from build123d import *

# Parameters (mm, degrees)
BOSS_EXTRU_1_DEPTH      = 39.5
ESQUISSE3_W             = 10
ESQUISSE3_H             = 5
ENL_V_MAT_EXTRU_1_DEPTH = 51.963222033
CUT_EXTRUDE1_DEPTH      = 64.947243881
CUT_EXTRUDE1_DEPTH_BACK = 64.947243881
SKETCH1_R               = 1.6
CUT_EXTRUDE2_DEPTH      = 51.963222033
FILLET1_R               = 5


with BuildPart() as part:
    # Esquisse1 → Boss.-Extru.1 (new body)
    with BuildSketch(Plane.XY):
        Polygon((-22, 0), (22, 0), (22, 15), (26, 15), (26, -4), (-26, -4), (-26, 15), (-22, 15), align=None)
    extrude(amount=BOSS_EXTRU_1_DEPTH)

    # Esquisse3 → Enlèv. mat.-Extru.1 (cut, through all)
    with BuildSketch(Plane.XZ.offset(4)):
        with Locations((0, 7)):
            Rectangle(ESQUISSE3_W, ESQUISSE3_H)
    extrude(amount=-ENL_V_MAT_EXTRU_1_DEPTH, mode=Mode.SUBTRACT)

    # Sketch1 → Cut-Extrude1 (cut, two sides: drawn at the far end of the back side and taken through both)
    with BuildSketch(Plane(origin=(-22, 0, 0), x_dir=(0, 0, -1), z_dir=(1, 0, 0)).offset(-CUT_EXTRUDE1_DEPTH_BACK)):
        with Locations((-19.75, 6)):
            Circle(SKETCH1_R)
    extrude(amount=CUT_EXTRUDE1_DEPTH + CUT_EXTRUDE1_DEPTH_BACK, mode=Mode.SUBTRACT)

    # Sketch2 → Cut-Extrude2 (cut, through all)
    with BuildSketch(Plane.XZ.offset(4)):
        with BuildLine():
            Line((-16.9, 30.226876468), (-16.9, 15.226876468))
            ThreePointArc((-16.9, 15.226876468), (-18.5, 13.626876468), (-20.1, 15.226876468))
            Line((-20.1, 15.226876468), (-20.1, 30.226876468))
            ThreePointArc((-20.1, 30.226876468), (-18.5, 31.826876468), (-16.9, 30.226876468))
        make_face()
        with BuildLine():
            Line((20.1, 30.226876468), (20.1, 15.226876468))
            ThreePointArc((20.1, 15.226876468), (18.5, 13.626876468), (16.9, 15.226876468))
            Line((16.9, 15.226876468), (16.9, 30.226876468))
            ThreePointArc((16.9, 30.226876468), (18.5, 31.826876468), (20.1, 30.226876468))
        make_face()
    extrude(amount=-CUT_EXTRUDE2_DEPTH, mode=Mode.SUBTRACT)

    # Fillet1
    fillet1_edges = [part.edges().sort_by_distance(p)[0] for p in [
        (26, -4, 19.75),
        (-26, -4, 19.75),
    ]]
    fillet(fillet1_edges, radius=FILLET1_R)


solid = part.part
Design review of the part built by this model. Coordinates are the model's own, in mm. A direction names the side the tool comes from. Coordinates: 2 decimals unless noted, no trailing zeros. Order: outer loops, then holes, each group sorted by start corner. A loop starts at its lowest first (then second) coordinate and runs counter-clockwise, first axis right, second up. Notation, with made-up numbers: (53, 17.25) -> (69, 17.25) arc R19 ccw to (69, 50.25) -> close; hole circle Ø8 at (47, 27.25). An arc over 180 degrees is marked (long way). Use one line per item in the form item = value. Start each with the question number.
(1) Add section C-C on x = 18.5. State the section outline as (y, z) points.
(2) Add section A-A on y = 9.25. State the section outline as (x, z) points, plus the area to 3 significant figures.
(3) The part is to be moulded in two halves that separate along Z. For faces 4 (the flat face through (16.9, -2, 23)), 5 (the flat face through (5, -2, 7)), 6 (the flat face through (-24, 15, 19)), say which applies: +Z half, -Z half, draft (parallel to the pull), parting line (faces both ways), or undercut.
(4) For faces 1 (the flat face through (0, -2, 9.5)), 2 (the flat face through (0, 0, 19)), 3 (the cylindrical face through (24, 5, 21)), list the 3-axis set-ups (+Z, -Z, +X, -X, +Y, -Y) from which the entire face can be reached by the end or side of a thin tool; tool diameter is ignored.
(5) Add section D-D on z = 26. State the section outline as (x, y) points.
(6) Insertion check: pin 1 (2 mm diameter, centred on y = -2, z = 22.5, fed in from -X); pin 2 (3 mm diameter, centred on y = -3, z = 24.5, fed in from +X); pin 3 (1 mm diameter, centred on x = 3, y = 1, fed in from +Z); pin 4 (3 mm diameter, centred on x = 16, z = 33, fed in from +Y). Each pin has a flat end and moves straight along its axis. Give the tip position at first contact, or say it passes through.
(7) Add section B-B on z = 19.75. State the section outline as (x, y) points, plus the area to 3 significant figures.
(8) For probe 1 along Z at (x, y) = (24.15, 6); probe 2 along X at (y, z) = (12, 34); probe 3 along X at (y, z) = (-2.75, 28), list the stretches that pass through material, from the lowest coordinate up.
Answer block:
q1.outline = (-4, 0) -> (0, 0) -> (0, 13.63) -> (-4, 13.63) -> close; (-4, 31.83) -> (0, 31.83) -> (0, 39.5) -> (-4, 39.5) -> close
q2.outline = (-26, 0) -> (-22, 0) -> (-22, 39.5) -> (-26, 39.5) -> close; (22, 0) -> (26, 0) -> (26, 39.5) -> (22, 39.5) -> close
q2.area = 316 mm²
q3.face_4 = undercut
q3.face_5 = undercut
q3.face_6 = draft
q4.face_1 = +Y, -Y
q4.face_2 = +Z, -Z, +Y
q4.face_3 = +X, -X
q5.outline = (-26, 1) arc R5 ccw to (-21, -4) -> (-20.1, -4) -> (-20.1, 0) -> (-22, 0) -> (-22, 15) -> (-26, 15) -> close; (-16.9, -4) -> (16.9, -4) -> (16.9, 0) -> (-16.9, 0) -> close; (20.1, -4) -> (21, -4) arc R5 ccw to (26, 1) -> (26, 15) -> (22, 15) -> (22, 0) -> (20.1, 0) -> close
q6.pin_1 = -25.58
q6.pin_2 = 25.33
q6.pin_3 = through
q6.pin_4 = 0
q7.outline = (-26, 1) arc R5 ccw to (-21, -4) -> (-20.1, -4) -> (-20.1, 0) -> (-22, 0) -> (-22, 4.4) -> (-26, 4.4) -> close; (-26, 7.6) -> (-22, 7.6) -> (-22, 15) -> (-26, 15) -> close; (-16.9, -4) -> (16.9, -4) -> (16.9, 0) -> (-16.9, 0) -> close; (20.1, -4) -> (21, -4) arc R5 ccw to (26, 1) -> (26, 4.4) -> (22, 4.4) -> (22, 0) -> (20.1, 0) -> close; (22, 7.6) -> (26, 7.6) -> (26, 15) -> (22, 15) -> close
q7.area = 266 mm²
q8.probe_1 = 0 to 18.15, 21.35 to 39.5
q8.probe_2 = -26 to -22, 22 to 26
q8.probe_3 = -24.31 to -20.1, -16.9 to 16.9, 20.1 to 24.31
